from build123d import *

# Parameters (mm, degrees)
SKETCH_1_W          = 67
SKETCH_1_H          = 42
EXTRUDE_1_DEPTH     = 6
SKETCH_2_R          = 2.25
CUT_EXTRUDE_1_DEPTH = 9
FILLET_1_R          = 6
SKETCH_3_R          = 12
SKETCH_3_R_2        = 1.8
CUT_EXTRUDE_2_DEPTH = 10
SKETCH_4_R          = 3.5
CUT_EXTRUDE_3_DEPTH = 2
SKETCH_8_R          = 4
SKETCH_8_R_2        = 2.25
CUT_EXTRUDE_6_DEPTH = 4
CUT_EXTRUDE_7_DEPTH = 26


with BuildPart() as part:
    # Sketch 1 → Extrude 1 (new body)
    with BuildSketch(Plane.XY):
        with Locations((33.5, 21)):
            Rectangle(SKETCH_1_W, SKETCH_1_H)
    extrude(amount=EXTRUDE_1_DEPTH)

    # Sketch 2 → Cut-Extrude 1 (cut)
    with BuildSketch(Plane(origin=(0, 0, 0), x_dir=(-1, 0, 0), z_dir=(0, 0, -1))):
        with Locations((-62, 6)):
            Circle(SKETCH_2_R)
        with Locations((-62, 33)):
            Circle(SKETCH_2_R)
        with Locations((-5, 6)):
            Circle(SKETCH_2_R)
        with Locations((-5, 33)):
            Circle(SKETCH_2_R)
    extrude(amount=-CUT_EXTRUDE_1_DEPTH, mode=Mode.SUBTRACT)

    # Fillet 1
    fillet_1_edges = [part.edges().sort_by_distance(p)[0] for p in [
        (0, 42, 3),
        (67, 42, 3),
        (67, 0, 3),
        (0, 0, 3),
    ]]
    fillet(fillet_1_edges, radius=FILLET_1_R)

    # Sketch 3 → Cut-Extrude 2 (cut)
    with BuildSketch(Plane(origin=(0, 0, 0), x_dir=(-1, 0, 0), z_dir=(0, 0, -1))):
        with Locations((-33.5, 21)):
            Circle(SKETCH_3_R)
        with Locations((-18, 36.5)):
            Circle(SKETCH_3_R_2)
        with Locations((-18, 5.5)):
            Circle(SKETCH_3_R_2)
        with Locations((-49, 5.5)):
            Circle(SKETCH_3_R_2)
        with Locations((-49, 36.5)):
            Circle(SKETCH_3_R_2)
    extrude(amount=-CUT_EXTRUDE_2_DEPTH, mode=Mode.SUBTRACT)

    # Sketch 4 → Cut-Extrude 3 (cut)
    with BuildSketch(Plane.XY.offset(6)):
        with Locations((18, 5.5)):
            Circle(SKETCH_4_R)
        with Locations((18, 36.5)):
            Circle(SKETCH_4_R)
        with Locations((49, 5.5)):
            Circle(SKETCH_4_R)
        with Locations((49, 36.5)):
            Circle(SKETCH_4_R)
    extrude(amount=-CUT_EXTRUDE_3_DEPTH, mode=Mode.SUBTRACT)

    # Sketch 8 → Cut-Extrude 6 (cut)
    with BuildSketch(Plane(origin=(0, 0, 0), x_dir=(-1, 0, 0), z_dir=(0, 0, -1))):
        with Locations((-44, 33)):
            Circle(SKETCH_8_R)
        with Locations((-44, 33)):
            Circle(SKETCH_8_R_2, mode=Mode.SUBTRACT)
    extrude(amount=-CUT_EXTRUDE_6_DEPTH, mode=Mode.SUBTRACT)

    # Sketch 8_2 → Cut-Extrude 7 (cut)
    with BuildSketch(Plane(origin=(0, 0, 0), x_dir=(-1, 0, 0), z_dir=(0, 0, -1))):
        with BuildLine():
            ThreePointArc((-46.25, 33), (-44, 30.75), (-41.75, 33))
            Line((-41.75, 33), (-46.25, 33))
        make_face()
        with BuildLine():
            Line((-46.25, 33), (-41.75, 33))
            ThreePointArc((-41.75, 33), (-44, 35.25), (-46.25, 33))
        make_face()
    extrude(amount=-CUT_EXTRUDE_7_DEPTH, mode=Mode.SUBTRACT)


solid = part.part
Geometry check sheet. Reference: the model listing, model coordinates, mm. A direction names the side the tool comes from. Coordinates: 2 decimals unless noted, no trailing zeros. Order: outer loops, then holes, each group sorted by start corner. A loop starts at its lowest first (then second) coordinate and runs counter-clockwise, first axis right, second up. Notation, with made-up numbers: (12.5, 30) -> (33.5, 30) arc R32 cw to (33.5, 68) -> close; hole circle Ø2 at (32.5, 79). An arc over 180 degrees is marked (long way). Use a Markdown table: item, result. Add a question column.
1. Set-up check for faces 4 (the face through (42, 31, 4)), 5 (the face through (27.963, 10.354, 2.958)), 6 (the face through (16, 6, 4)): record each of +Z, -Z, +X, -X, +Y, -Y from which the full face is reachable in a straight line by a thin tool's end or side.
2. Material ranges on L1, parallel to Y at x = 49, z = 1.95; L2, parallel to Y at x = 44, z = 1.9; L3, parallel to X at y = 31, z = 3.9, recorded low to high.
3. Cross-section at D-D (z = 0.7). Give the number of separate pieces and of enclosed holes in the cut face, and give its area (3 significant figures).
4. Mould release check, pull along X, two halves, no side actions. Record for faces 1 (the face through (33, 0, 3)), 2 (the face through (18.234, 38.285, 1.972)), 3 (the face through (1.711, 40.196, 3.042)): pulls with the +X half, pulls with the -X half, needs draft (parallel to the pull), parting line crosses it, or undercut.
5. Cross-section at A-A (x = 33.5). Enter the section's corners in (y, z).
6. Cross-section at B-B (y = 21). Enter the section's corners in (x, z).
7. Go/stop test with flat-tipped pins: pin 1 Ø4 at (x, y) = (62, 6) entering from -Z; pin 2 Ø6 at (x, y) = (44, 33) entering from -Z; pin 3 Ø5.5 at (x, y) = (47.5, 4) entering from +Z; pin 4 Ø6 at (x, y) = (49, 5.5) entering from +Z. Record where each tip stops, or that it passes through.
8. Cross-section at C-C (x = 49). Enter the section's corners in (y, z).
Filled sheet:
| question | item | result |
|---|---|---|
| 1 | face 4 | -Z |
| 1 | face 5 | +Z, -Z |
| 1 | face 6 | +Z |
| 2 | L1 | 0 to 3.7, 7.3 to 34.7, 38.3 to 42 |
| 2 | L2 | 0 to 15.19, 26.81 to 29, 37 to 42 |
| 2 | L3 | 0 to 3.97, 6.03 to 26.87, 40.13 to 40.54, 47.46 to 60.97, 63.03 to 67 |
| 3 | separate pieces | 1 |
| 3 | enclosed holes | 9 |
| 3 | area | 2,180 mm2 |
| 4 | face 1 | needs draft |
| 4 | face 2 | undercut |
| 4 | face 3 | pulls with the -X half |
| 5 | outline | (0, 0) -> (9, 0) -> (9, 6) -> (0, 6) -> close; (33, 0) -> (42, 0) -> (42, 6) -> (33, 6) -> close |
| 6 | outline | (0, 0) -> (21.5, 0) -> (21.5, 6) -> (0, 6) -> close; (45.5, 0) -> (67, 0) -> (67, 6) -> (45.5, 6) -> close |
| 7 | pin 1 | through |
| 7 | pin 2 | z = 4 |
| 7 | pin 3 | z = 6 |
| 7 | pin 4 | z = 4 |
| 8 | outline | (0, 0) -> (3.7, 0) -> (3.7, 4) -> (2, 4) -> (2, 6) -> (0, 6) -> close; (7.3, 0) -> (34.7, 0) -> (34.7, 4) -> (33, 4) -> (33, 6) -> (9, 6) -> (9, 4) -> (7.3, 4) -> close; (38.3, 0) -> (42, 0) -> (42, 6) -> (40, 6) -> (40, 4) -> (38.3, 4) -> close |
